Verification items for the finished model (mm, model axes). A direction names the side the tool comes from. Give positions to 0.01 mm unless a question says otherwise; leave off trailing zeros. Order: outer loops, then holes, each group sorted by start corner. A loop starts at its lowest first (then second) coordinate and runs counter-clockwise, first axis right, second up. Notation, with made-up numbers: (8.5, 63) -> (15.5, 63) arc R25 ccw to (15.5, 83) -> close; hole circle Ø6 at (70.5, -19.75). An arc over 180 degrees is marked (long way). Write each question's results on one line, items separated by ' | '. Start each with the question number.
1. Cross-section at C-C, the plane z = -57.15. Enter the section's corners in (x, y), then the cut area to 3 significant figures.
2. Cross-section at D-D, the plane x = 57.15. Enter the section's corners in (y, z), then the cut area to 3 significant figures.
3. Cross-section at A-A, the plane x = 152.4. Enter the section's corners in (y, z) (3 decimals), then the cut area to 3 significant figures.
4. Material ranges on L1, parallel to X at y = 2.75, z = -57.15; L2, parallel to Z at x = 19.05, y = 2.25; L3, parallel to X at y = 3.25, z = -19.05, recorded low to high. Write a range as from..to.
5. Depth check by flat-ended pin: pin 1 Ø7.5 at (x, z) = (152.4, -130.15) entering from -Y. Enter the tip coordinate at first touch or a pass-through.
6. Set-up check for faces 5 (the face through (125, 3, 0)), 6 (the face through (210.253, 3.219, -216.359)): record each of +Z, -Z, +X, -X, +Y, -Y from which the full face is reachable in a straight line by a thin tool's end or side.
7. Cross-section at B-B, the plane z = -88.9. Enter the section's corners in (x, y), then the cut area to 3 significant figures.
8. Mould release check, pull along X, two halves, no side actions. Record for faces 1 (the face through (61.313, 3.131, -89.083)), 2 (the face through (254, 3, -125)), 3 (the face through (0, 3, -125)), 4 (the face through (61.313, 3.131, -228.783)): +X half, -X half, draft (parallel to the pull), parting line (faces both ways), or undercut.
from build123d import *

# Parameters (mm, degrees)
SKETCH1_W                        = 254
SKETCH1_H                        = 254
BOSS_EXTRUDE1_DEPTH              = 6.35
F_3_4_0_75_DIAMETER_HOLE1_D      = 19.05
F_3_8_0_375_DIAMETER_HOLE1_D     = 9.525
F_21_64_0_32813_DIAMETER_HOLE1_D = 8.334502
LPATTERN1_COUNT                  = 2
LPATTERN1_PITCH                  = 38.1
LPATTERN1_COUNT_DIR2             = 4
LPATTERN1_PITCH_DIR2             = 69.85
F_21_64_0_32813_DIAMETER_HOLE2_D = 8.334502
LPATTERN2_COUNT                  = 2
LPATTERN2_PITCH                  = 38.1
LPATTERN2_COUNT_DIR2             = 3
LPATTERN2_PITCH_DIR2             = 69.85
CUT_EXTRUDE1_DEPTH               = 360.266367059
FILLET1_R                        = 3.175


with BuildPart() as part:
    # Sketch1 → Boss-Extrude1 (new body)
    with BuildSketch(Plane(origin=(0, 0, 0), x_dir=(1, 0, 0), z_dir=(0, 1, 0))):
        with Locations((127, 127)):
            Rectangle(SKETCH1_W, SKETCH1_H)
    extrude(amount=BOSS_EXTRUDE1_DEPTH)

    # 3/4 (0.75) Diameter Hole1 (through all)
    with Locations(Plane(origin=(0, 6.35, 0), x_dir=(1, 0, 0), z_dir=(0, 1, 0))):
        with Locations((152.4, 152.4)):
            Hole(F_3_4_0_75_DIAMETER_HOLE1_D / 2)

    # 3/8 (0.375) Diameter Hole1 (through all)
    with Locations(Plane(origin=(0, 6.35, 0), x_dir=(1, 0, 0), z_dir=(0, 1, 0))):
        with Locations((152.4, 174.6504), (152.4, 130.1496)):
            Hole(F_3_8_0_375_DIAMETER_HOLE1_D / 2)

    # 21/64 (0.32813) Diameter Hole1 (through all)
    with Locations(Plane(origin=(0, 6.35, 0), x_dir=(1, 0, 0), z_dir=(0, 1, 0))):
        with Locations((19.05, 19.05)):
            f_21_64_0_32813_diameter_hole1 = Hole(F_21_64_0_32813_DIAMETER_HOLE1_D / 2)

    # LPattern1: 21_64 _0.32813_ Diameter Hole1 2 × 4
    with Locations(*[(i * LPATTERN1_PITCH, 0, -j * LPATTERN1_PITCH_DIR2) for i in range(LPATTERN1_COUNT) for j in range(LPATTERN1_COUNT_DIR2) if (i, j) != (0, 0)]):
        add(f_21_64_0_32813_diameter_hole1, mode=Mode.SUBTRACT)

    # 21/64 (0.32813) Diameter Hole2 (through all)
    with Locations(Plane(origin=(0, 6.35, 0), x_dir=(1, 0, 0), z_dir=(0, 1, 0))):
        with Locations((234.95, 19.05)):
            f_21_64_0_32813_diameter_hole2 = Hole(F_21_64_0_32813_DIAMETER_HOLE2_D / 2)

    # LPattern2: 21_64 _0.32813_ Diameter Hole2 2 × 3
    with Locations(*[(-j * LPATTERN2_PITCH_DIR2, 0, -i * LPATTERN2_PITCH) for i in range(LPATTERN2_COUNT) for j in range(LPATTERN2_COUNT_DIR2) if (i, j) != (0, 0)]):
        add(f_21_64_0_32813_diameter_hole2, mode=Mode.SUBTRACT)

    # Sketch10 → Cut-Extrude1 (cut, through all)
    with BuildSketch(Plane(origin=(0, 6.35, 0), x_dir=(1, 0, 0), z_dir=(0, 1, 0))):
        Polygon((188.084920071, 194.191494234), (232.986200677, 239.092774839), (239.092774839, 232.986200677), (194.191494234, 188.084920071), align=None)
    extrude(amount=-CUT_EXTRUDE1_DEPTH, mode=Mode.SUBTRACT)

    # Fillet1
    fillet1_edges = [part.edges().sort_by_distance(p)[0] for p in [
        (194.191494234, 3.175, -188.084920071),
        (188.084920071, 3.175, -194.191494234),
        (232.986200677, 3.175, -239.092774839),
        (239.092774839, 3.175, -232.986200677),
    ]]
    fillet(fillet1_edges, radius=FILLET1_R)


solid = part.part
Results below:
1) outline: (0, 0) -> (91.08, 0) -> (91.08, 6.35) -> (0, 6.35) -> close; (99.42, 0) -> (160.93, 0) -> (160.93, 6.35) -> (99.42, 6.35) -> close; (169.27, 0) -> (230.78, 0) -> (230.78, 6.35) -> (169.27, 6.35) -> close; (239.12, 0) -> (254, 0) -> (254, 6.35) -> (239.12, 6.35) -> close | area: 1,450 mm²
2) outline: (0, -254) -> (6.35, -254) -> (6.35, -232.77) -> (0, -232.77) -> close; (0, -224.43) -> (6.35, -224.43) -> (6.35, -162.92) -> (0, -162.92) -> close; (0, -154.58) -> (6.35, -154.58) -> (6.35, -93.07) -> (0, -93.07) -> close; (0, -84.73) -> (6.35, -84.73) -> (6.35, -23.22) -> (0, -23.22) -> close; (0, -14.88) -> (6.35, -14.88) -> (6.35, 0) -> (0, 0) -> close | area: 1,400 mm²
3) outline: (0, -254) -> (6.35, -254) -> (6.35, -179.413) -> (0, -179.413) -> close; (0, -169.888) -> (6.35, -169.888) -> (6.35, -161.925) -> (0, -161.925) -> close; (0, -142.875) -> (6.35, -142.875) -> (6.35, -134.912) -> (0, -134.912) -> close; (0, -125.387) -> (6.35, -125.387) -> (6.35, 0) -> (0, 0) -> close | area: 1,370 mm²
4) L1: x = 0..91.08, 99.42..160.93, 169.27..230.78, 239.12..254 | L2: z = -254..-232.77, -224.43..-162.92, -154.58..-93.07, -84.73..-23.22, -14.88..0 | L3: x = 0..14.88, 23.22..52.98, 61.32..91.08, 99.42..160.93, 169.27..230.78, 239.12..254
5) pin 1: passes through
6) face 5: +Z, +X, -X, +Y, -Y | face 6: +Y, -Y
7) outline: (0, 0) -> (14.88, 0) -> (14.88, 6.35) -> (0, 6.35) -> close; (23.22, 0) -> (52.98, 0) -> (52.98, 6.35) -> (23.22, 6.35) -> close; (61.32, 0) -> (254, 0) -> (254, 6.35) -> (61.32, 6.35) -> close | area: 1,510 mm²
8) face 1: undercut | face 2: +X half | face 3: -X half | face 4: undercut
